```python
from build123d import *

# Parameters (mm, degrees)
SKETCH1_R           = 73.025
BOSS_EXTRUDE1_DEPTH = 3.175
SKETCH2_R           = 3.175
CUT_EXTRUDE1_DEPTH  = 4.175
SKETCH3_R           = 40.64
CUT_EXTRUDE2_DEPTH  = 4.175


with BuildPart() as part:
    # Sketch1 → Boss-Extrude1 (new body)
    with BuildSketch(Plane(origin=(0, 0, 0), x_dir=(1, 0, 0), z_dir=(0, 1, 0))):
        Circle(SKETCH1_R)
    extrude(amount=BOSS_EXTRUDE1_DEPTH)

    # Sketch2 → Cut-Extrude1 (cut, through all)
    with BuildSketch(Plane(origin=(0, 3.175, 0), x_dir=(1, 0, 0), z_dir=(0, 1, 0))):
        with Locations((63.5, 0)):
            Circle(SKETCH2_R)
        with Locations((54.99261314, -31.75)):
            Circle(SKETCH2_R)
        with Locations((31.75, -54.99261314)):
            Circle(SKETCH2_R)
        with Locations((0, -63.5)):
            Circle(SKETCH2_R)
        with Locations((-31.75, -54.99261314)):
            Circle(SKETCH2_R)
        with Locations((-54.99261314, -31.75)):
            Circle(SKETCH2_R)
        with Locations((-63.5, 0)):
            Circle(SKETCH2_R)
        with Locations((-54.99261314, 31.75)):
            Circle(SKETCH2_R)
        with Locations((-31.75, 54.99261314)):
            Circle(SKETCH2_R)
        with Locations((0, 63.5)):
            Circle(SKETCH2_R)
        with Locations((31.75, 54.99261314)):
            Circle(SKETCH2_R)
        with Locations((54.99261314, 31.75)):
            Circle(SKETCH2_R)
    extrude(amount=-CUT_EXTRUDE1_DEPTH, mode=Mode.SUBTRACT)

    # Sketch3 → Cut-Extrude2 (cut, through all)
    with BuildSketch(Plane(origin=(0, 3.175, 0), x_dir=(1, 0, 0), z_dir=(0, 1, 0))):
        Circle(SKETCH3_R)
    extrude(amount=-CUT_EXTRUDE2_DEPTH, mode=Mode.SUBTRACT)


solid = part.part
```
The listing builds one solid part. Answer for the finished solid, in the listing's coordinates (mm). Coordinates: 2 decimals unless noted, no trailing zeros. Loops run counter-clockwise (first coordinate to the right, second up) from the corner with the lowest first, then second, coordinate; pieces in that order, holes last. Notation, with made-up numbers: (75, -35.75) -> (127, -35.75) arc R24 ccw to (127, -8.75) -> close; hole circle Ø8 at (81.5, 70.25). An arc over 180 degrees is marked (long way). Use one line per item in the form item = value. Start each with the question number.
Item 1: The mould has two halves that part along X. Classify faces 1 (the face through (31.337, 1.61, 51.845)), 2 (the face through (31, 0, 31)), 3 (the face through (69.653, 1.565, -21.935)): released by +X, released by -X, zero draft, split by the parting line, or undercut.
Item 2: The part is cut by section D-D on y = 2.6. Count the separate pieces of the cut face and the enclosed holes in it, then the cut area to 3 significant figures.
Item 3: The part is cut by section C-C on x = -15. Determine the outline of the cut face in (y, z) (3 decimals).
Item 4: Flat-ended cylindrical pins translate along their axes: pin 1 Ø5.5 at (x, z) = (63.5, 0) entering from +Y; pin 2 Ø1 at (y, z) = (1, -50.5) entering from -X. Find the tip coordinate at first contact, or state that the pin passes through.
Item 5: Consider L1, parallel to Z at x = 0, y = 1.3 (3 decimals); L2, parallel to X at y = 1.6, z = 31.75. Determine where each line is inside the solid, lowest interval first. Write a range as [from, to].
Item 6: The part is cut by section B-B on z = 7. Determine the outline of the cut face in (x, y) (3 decimals), then the cut area to 3 significant figures.
Item 7: The part is cut by section A-A on x = 0. Determine the outline of the cut face in (y, z) (3 decimals).
Answer key:
q1.face_1 = undercut
q1.face_2 = zero draft
q1.face_3 = split by the parting line
q2.separate_pieces = 1
q2.enclosed_holes = 13
q2.area = 11,200 mm2
q3.outline = (0, -71.468) -> (3.175, -71.468) -> (3.175, -37.77) -> (0, -37.77) -> close; (0, 37.77) -> (3.175, 37.77) -> (3.175, 71.468) -> (0, 71.468) -> close
q4.pin_1 = through
q4.pin_2 = -53.22
q5.L1 = [-73.025, -66.675], [-60.325, -40.64], [40.64, 60.325], [66.675, 73.025]
q5.L2 = [-65.76, -58.17], [-51.82, -25.37], [25.37, 51.82], [58.17, 65.76]
q6.outline = (-72.689, 0) -> (-40.033, 0) -> (-40.033, 3.175) -> (-72.689, 3.175) -> close; (40.033, 0) -> (72.689, 0) -> (72.689, 3.175) -> (40.033, 3.175) -> close
q6.area = 207 mm2
q7.outline = (0, -73.025) -> (3.175, -73.025) -> (3.175, -66.675) -> (0, -66.675) -> close; (0, -60.325) -> (3.175, -60.325) -> (3.175, -40.64) -> (0, -40.64) -> close; (0, 40.64) -> (3.175, 40.64) -> (3.175, 60.325) -> (0, 60.325) -> close; (0, 66.675) -> (3.175, 66.675) -> (3.175, 73.025) -> (0, 73.025) -> close
